Autodesk Inventor part; units mm, degrees
ref_plane "Work Plane1" through (-1.8331, 3.175, 83.0707) normal (0.866, 0.5, 0) x (0, 0, -1)
ref_plane "YZ Plane" through (0, 0, 0) normal (1, 0, 0) x (0, 1, 0)
ref_plane "XZ Plane" through (0, 0, 0) normal (0, 1, 0) x (-1, 0, 0)
sketch "Sketch1" plane through (0, 0, 0) normal (0, 0, 1) x (1, 0, 0)
  line L0 (-3.6662, 6.35) -> (3.6662, 6.35)
  line L1 (3.6662, 6.35) -> (7.3323, 0)
  line L2 (7.3323, 0) -> (3.6662, -6.35)
  line L3 (3.6662, -6.35) -> (-3.6662, -6.35)
  line L4 (-3.6662, -6.35) -> (-7.3323, 0)
  line L5 (-7.3323, 0) -> (-3.6662, 6.35)
  point P0 (0, 0)
  point P1 (0, 0)
  dimension "d0" = 7.3323
extrude "Extrusion1" add sketch "Sketch1" along normal mid plane 166.1414
sketch "Sketch2" plane through (0, 0, -83.0707) normal (0, 0, -1) x (-1, 0, 0)
  circle A0 centre (0, 0) radius 3.175
  circle A1 centre (0, 0) radius 6.35
  dimension "d3" = 6.35
  dimension "d4" = 12.7
extrude "Extrusion2" add sketch "Sketch2" along normal blind 6.35
chamfer "Chamfer1" distance 0.7874 angle 45 1 edges at (6.35, 0, -89.4207)
ref_plane "Work Plane1" through (-1.8331, 3.175, 83.0707) normal (0.866, 0.5, 0) x (0, 0, -1)
sketch "Sketch3" plane through (-1.8331, 3.175, 83.0707) normal (0.866, 0.5, 0) x (0, 0, -1)
  line L0 (166.1414, -3.6662) -> (166.1414, 0)
  line L1 (154.432, 1.9218) -> (154.432, 5.7318)
  line L2 (152.8445, 1.9218) -> (152.8445, 5.7318)
  line L3 (154.432, 1.9218) -> (159.062, 1.9218) construction
  line L4 (166.1414, -3.6662) -> (163.6991, -3.6662)
  line L5 (154.432, 5.7318) -> (152.8445, 5.7318)
  line L6 (154.432, 1.9218) -> (152.8445, 1.9218)
  point P0 (83.0707, -3.6662)
  dimension "d10" = 11.7094
  dimension "d11" = 1.5875
  dimension "d12" = 5.588
  dimension "d13" = 3.81
revolve "Revolution1" cut sketch "Sketch3" angle 360 about axis through (0, 0, -83.0707) along (0, 0, 1)
properties part number "Gearbox_hex_shaft"
Work out the finished part from the listing and answer in its coordinate system (mm). A direction names the side the tool comes from. Give positions to 0.01 mm unless a question says otherwise; leave off trailing zeros. Loops run counter-clockwise (first coordinate to the right, second up) from the corner with the lowest first, then second, coordinate; pieces in that order, holes last. Notation, with made-up numbers: (-19, 3.25) - (12, 3.25) arc R7 ccw to (12, 10.25) - close; hole circle Ø11 at (11.25, 51). An arc over 180 degrees is marked (long way). Answer in a Markdown table with one row per item.
(1) Flat-ended cylindrical pins translate along their axes: pin 1 Ø0.9 at (x, y) = (-6.5, 1) entering from -Z; pin 2 Ø0.5 at (x, y) = (6.5, 1.5) entering from -Z; pin 3 Ø6 at (y, z) = (4, 48.5) entering from -X. Find the tip coordinate at first contact, or state that the pin passes through.
Results list:
| item | result |
|---|---|
| pin 1 | stops at z = -88.86 |
| pin 2 | stops at z = -83.07 |
| pin 3 | stops at x = -6.75 |
(2) For a pull along Y with two mould halves and no side action, classify faces 1 (the face through (-5.474, -3.219, -77.298)), 2 (the face through (0, 0, -83.071)), 3 (the face through (1.38, 6.2, -85.81)), 4 (the face through (-5.525, 3.131, -77.298)) as pulls with the +Y half, pulls with the -Y half, needs draft (parallel to the pull), parting line crosses it, or undercut.
Results list:
| item | result |
|---|---|
| face 1 | pulls with the -Y half |
| face 2 | undercut |
| face 3 | parting line crosses it |
| face 4 | pulls with the +Y half |
(3) Section A-A (z = 6) is taken. Give the vertices of the cut face in (x, y).
Results list:
| item | result |
|---|---|
| outline | (-7.33, 0) - (-3.67, -6.35) - (3.67, -6.35) - (7.33, 0) - (3.67, 6.35) - (-3.67, 6.35) - close |
(4) A tool of negligible diameter and unlimited length cuts with its end or side. For faces 5 (the face through (-3, 6, -83.071)), 6 (the face through (3, -6, -83.071)), 7 (the face through (3, 6, -83.071)), 8 (the face through (-5, 3, -69.774)), from which of +Z, -Z, +X, -X, +Y, -Y can it reach the whole face along a straight path? Write none if from no direction.
Results list:
| item | result |
|---|---|
| face 5 | -Z, -X, +Y |
| face 6 | -Z, +X, -Y |
| face 7 | -Z, +X, +Y |
| face 8 | none |
(5) Consider L1, parallel to Y at x = 0, z = -87 (3 decimals); L2, parallel to Z at x = 2.75, y = -6; L3, parallel to Z at x = -0.25, y = 1. Determine where each line is inside the solid, lowest interval first. Write a range as [from, to].
Results list:
| item | result |
|---|---|
| L1 | y = [-6.35, -3.175], [3.175, 6.35] |
| L2 | z = [-83.07, -71.36], [-69.77, 83.07] |
| L3 | z = [-83.07, 83.07] |
